Here's how the part is built. I have some questions about the finished solid (model axes, mm). Round coordinates to 2 decimals unless told otherwise and drop trailing zeros. Loops run counter-clockwise (first coordinate to the right, second up) from the corner with the lowest first, then second, coordinate; pieces in that order, holes last. Notation, with made-up numbers: M -5.75,13 L 32.25,13 A19 cw 32.25,47 Z; hole C 75.5,71.25 d4. An arc over 180 degrees is marked long. Answer as a JSON object with one key per item and string values.
from build123d import *

# Parameters (mm, degrees)
F0_W     = 10
F0_H     = 10
F1_DEPTH = 120
F3_D     = 3.4


with BuildPart() as f1:
    # F0 (on Front) → F1 (new body)
    with BuildSketch(Plane.XZ):
        Rectangle(F0_W, F0_H)
    extrude(amount=F1_DEPTH)

    # F3 (through all)
    with Locations(Plane.XY.offset(5)):
        with Locations((0, -10), (0, -110)):
            Hole(F3_D / 2)


solid = f1.part
Item 1: I want a section at B-B on x = 0. List the corners of the cut face in (y, z) for me.
Solution:
{"outline": "M -120,-5 L -111.7,-5 L -111.7,5 L -120,5 Z; M -108.3,-5 L -11.7,-5 L -11.7,5 L -108.3,5 Z; M -8.3,-5 L 0,-5 L 0,5 L -8.3,5 Z"}
Item 2: If I drill on L1, parallel to Y at x = 0, z = 2.25; L2, parallel to X at y = -110, z = 2.75; L3, parallel to Y at x = -1, z = -3, over which ranges is the centre line in solid material (lowest first)? Write a range as from..to.
Solution:
{"L1": "y = -120..-111.7, -108.3..-11.7, -8.3..0", "L2": "x = -5..-1.7, 1.7..5", "L3": "y = -120..-111.37, -108.63..-11.37, -8.63..0"}
Item 3: We'd pull the mould along X, two halves only. Please class faces 1 (the face through (0.37, -111.66, -0.07)), 2 (the face through (0.37, -11.66, -0.07)), 3 (the face through (0, -59, -5)), 4 (the face through (5, -59, 0)): +X half, -X half, draft (parallel to the pull), parting line (faces both ways), or undercut.
Solution:
{"face 1": "undercut", "face 2": "undercut", "face 3": "draft", "face 4": "+X half"}
Item 4: I want a section at A-A on y = -10. List the corners of the cut face in (x, z) for me.
Solution:
{"outline": "M -5,-5 L -1.7,-5 L -1.7,5 L -5,5 Z; M 1.7,-5 L 5,-5 L 5,5 L 1.7,5 Z"}
Item 5: I want a section at C-C on z = -2. List the corners of the cut face in (x, y) for me.
Solution:
{"outline": "M -5,-120 L 5,-120 L 5,0 L -5,0 Z; hole C 0,-110 d3.4; hole C 0,-10 d3.4"}
